The model under review builds one solid part; all positions refer to its coordinate system, in mm. Give positions to 0.01 mm unless a question says otherwise; leave off trailing zeros. Write each loop counter-clockwise with the first axis right and the second up, starting at its lowest first coordinate (ties: lowest second). Pieces come first, ordered by that corner, then holes. Notation, with made-up numbers: (58.25, 78.25) -> (82.25, 78.25) arc R20 cw to (82.25, 105.25) -> close; hole circle Ø5 at (80.5, 5). An arc over 180 degrees is marked (long way). Use CSV: the item, a comma, the result in double quotes.
Autodesk Inventor part; units mm, degrees
ref_plane "YZ Plane" through (0, 0, 0) normal (1, 0, 0) x (0, 1, 0)
ref_plane "XZ Plane" through (0, 0, 0) normal (0, 1, 0) x (-1, 0, 0)
ref_plane "XY Plane" through (0, 0, 0) normal (0, 0, 1) x (1, 0, 0)
sketch "Sketch1" plane through (0, 0, 0) normal (0, 1, 0) x (-1, 0, 0)
  line L0 (0, 0) -> (-93, 0)
  line L1 (-93, 0) -> (-93, 20)
  line L2 (-93, 20) -> (0, 20)
  line L3 (0, 20) -> (0, 0)
  dimension "d0" = 93
  dimension "d1" = 20
extrude "Extrusion1" add sketch "Sketch1" along normal blind 2
hole "Hole1" at (6.8497, 2, 9.7688) direction (0, -1, 0) diameter 5.5 end through all
pattern_linear "Rectangular Pattern1" count 3 spacing 40 along (1, 0, 0) of "Hole1"
properties part number "flatbarx2" material "Aluminum 6061"
Q1. Consider section B-B (y = 0.6). Write out the cut boundary in (x, z).
Derived:
outline,"(0, 0) -> (93, 0) -> (93, 20) -> (0, 20) -> close; hole circle Ø5.5 at (6.85, 9.77); hole circle Ø5.5 at (46.85, 9.77); hole circle Ø5.5 at (86.85, 9.77)"
Q2. The part is to be moulded in two halves that separate along Z. For faces 1 (the flat face through (47, 0, 15)), 2 (the cylindrical face through (49.534, 0.986, 9.173)), 3 (the flat face through (46, 1, 0)), say which applies: pulls with the +Z half, pulls with the -Z half, needs draft (parallel to the pull), parting line crosses it, or undercut.
Derived:
face 1,"needs draft"
face 2,"undercut"
face 3,"pulls with the -Z half"
Q3. To check wall thickness, follow probe 1 along X at (y, z) = (0.7, 12); probe 2 along Z at (x, y) = (44.5, 0.35); probe 3 along Z at (x, y) = (46.5, 1.3). State the ranges of each line that lie inside material, in increasing order.
Derived:
probe 1,"x = 0 to 5.24, 8.46 to 45.24, 48.46 to 85.24, 88.46 to 93"
probe 2,"z = 0 to 8.34, 11.2 to 20"
probe 3,"z = 0 to 7.04, 12.5 to 20"
Q4. Consider section A-A (z = 10.5). Write out the cut boundary in (x, y).
Derived:
outline,"(0, 0) -> (4.2, 0) -> (4.2, 2) -> (0, 2) -> close; (9.5, 0) -> (44.2, 0) -> (44.2, 2) -> (9.5, 2) -> close; (49.5, 0) -> (84.2, 0) -> (84.2, 2) -> (49.5, 2) -> close; (89.5, 0) -> (93, 0) -> (93, 2) -> (89.5, 2) -> close"
